Autodesk Inventor part; units mm, degrees
ref_plane "YZ Plane" through (0, 0, 0) normal (1, 0, 0) x (0, 1, 0)
ref_plane "XZ Plane" through (0, 0, 0) normal (0, 1, 0) x (-1, 0, 0)
ref_plane "XY Plane" through (0, 0, 0) normal (0, 0, 1) x (1, 0, 0)
sketch "スケッチ1" plane through (0, 0, 0) normal (0, 0, 1) x (1, 0, 0)
  circle A0 centre (-137.47813, 108.715013) radius 1.5
  circle A1 centre (-137.47813, 108.715013) radius 4
  circle A2 centre (-84.833891, 108.084965) radius 1.5
  circle A3 centre (-84.833891, 108.084965) radius 4
  arc A4 (-118.947299, 71.123436) -> (-117.73095, 71.382243) centre (-118.502117, 72.018876) ccw
  arc A5 (-114.600271, 73.907195) -> (-117.73095, 71.382243) centre (-110, 65) ccw
  arc A6 (-114.600271, 73.907195) -> (-114.089743, 75.041147) centre (-115.059151, 74.795694) ccw
  line L0 (-114.089743, 75.041147) -> (-119.33341, 95.750821)
  arc A7 (-119.33341, 95.750821) -> (-120.080809, 96.480412) centre (-120.302818, 95.505368) ccw
  arc A8 (-121.730917, 97.23053) -> (-120.080809, 96.480412) centre (-119.081767, 100.868113) ccw
  arc A9 (-121.730917, 97.23053) -> (-122.772044, 97.31398) centre (-122.319616, 96.422178) ccw
  line L1 (-122.772044, 97.31398) -> (-145.176978, 85.94755)
  arc A10 (-145.176978, 85.94755) -> (-145.169733, 84.160308) centre (-144.724551, 85.055748) ccw
  line L2 (-145.169733, 84.160308) -> (-118.947299, 71.123436)
  arc A11 (-111.181518, 75.777506) -> (-110.19287, 75.023145) centre (-110.212109, 76.022959) ccw
  arc A12 (-100.681376, 68.696468) -> (-110.19287, 75.023145) centre (-110, 65) ccw
  arc A13 (-100.681376, 68.696468) -> (-99.603497, 68.076257) centre (-99.751838, 69.065193) ccw
  line L3 (-99.603497, 68.076257) -> (-77.042446, 71.460414)
  arc A14 (-77.042446, 71.460414) -> (-76.670938, 73.303609) centre (-77.190786, 72.449351) ccw
  line L4 (-76.670938, 73.303609) -> (-114.637331, 96.407596)
  arc A15 (-114.637331, 96.407596) -> (-116.126588, 95.307885) centre (-115.15718, 95.553338) ccw
  line L5 (-116.126588, 95.307885) -> (-111.181518, 75.777506)
  circle A16 centre (-150.294817, 85.033166) radius 1.5
  arc A17 (-124.129325, 99.989384) -> (-123.581755, 100.878808) centre (-124.581752, 100.881185) ccw
  arc A18 (-114.594354, 100.531773) -> (-123.581755, 100.878808) centre (-119.081767, 100.868113) ccw
  arc A19 (-114.594354, 100.531773) -> (-114.117, 99.602773) centre (-113.597151, 100.457031) ccw
  line L6 (-114.117, 99.602773) -> (-73.405222, 74.828115)
  arc A20 (-73.405222, 74.828115) -> (-72.36076, 74.831033) centre (-72.885373, 75.682374) ccw
  arc A21 (-73.660486, 68.382589) -> (-72.36076, 74.831033) centre (-70, 71) ccw
  arc A22 (-73.660486, 68.382589) -> (-74.622268, 68.789879) centre (-74.473928, 67.800942) ccw
  line L7 (-74.622268, 68.789879) -> (-99.158476, 65.109447)
  arc A23 (-99.158476, 65.109447) -> (-100.006948, 64.200283) centre (-99.010135, 64.120511) ccw
  arc A24 (-119.754961, 67.311137) -> (-100.006948, 64.200283) centre (-110, 65) ccw
  arc A25 (-119.754961, 67.311137) -> (-120.282843, 68.437115) centre (-120.728025, 67.541674) ccw
  line L8 (-120.282843, 68.437115) -> (-147.085218, 81.762313)
  arc A26 (-147.085218, 81.762313) -> (-148.083283, 81.700131) centre (-147.5304, 80.866873) ccw
  arc A27 (-148.11038, 88.384022) -> (-148.083283, 81.700131) centre (-150.294817, 85.033166) ccw
  arc A28 (-148.11038, 88.384022) -> (-147.111844, 88.329935) centre (-147.564271, 89.221736) ccw
  line L9 (-147.111844, 88.329935) -> (-124.129325, 99.989384)
  circle A29 centre (-110, 65) radius 7.025
  circle A30 centre (-119.081767, 100.868113) radius 1.5
  circle A31 centre (-70, 71) radius 1.5
  line L10 (-330.399972, 95) -> (-110, 65)
  circle A32 centre (-156.443214, 91.162336) radius 4
  circle A33 centre (-136.470623, 92.209055) radius 4
  line L11 (0, 0) -> (-155.794817, 0)
  line L12 (-329.051247, 104.90863) -> (-108.651275, 74.90863)
  circle A34 centre (-156.443214, 91.162336) radius 9
  circle A35 centre (-136.470623, 92.209055) radius 6
  line L13 (-156.443214, 91.162336) -> (-136.470623, 92.209055)
  circle A36 centre (-110, 65) radius 65
  circle A37 centre (-191.443214, 91.162336) radius 5
  line L14 (-191.443214, 91.162336) -> (-156.443214, 91.162336)
  line L15 (-191.443214, 91.162336) -> (-206.443214, 91.162336)
  circle A38 centre (-206.443214, 91.162336) radius 5
  line L16 (-206.443214, 91.162336) -> (-221.443214, 91.162336)
  circle A39 centre (-221.443214, 91.162336) radius 5
  line L17 (-221.443214, 91.162336) -> (-236.443214, 91.162336)
  circle A40 centre (-236.443214, 91.162336) radius 5
  line L18 (-206.843214, 96.14631) -> (-157.163214, 100.133489)
  line L19 (-206.843214, 86.178361) -> (-157.163214, 82.191182)
  line L20 (-135.882319, 98.180143) -> (-155.560758, 100.118968)
  line L21 (-154.629369, 82.34701) -> (-135.261393, 86.332171)
  circle A41 centre (-206.443214, 91.162336) radius 1.5
  circle A42 centre (-191.443214, 91.162336) radius 1.5
  line L22 (-236.443214, 91.162336) -> (-191.443214, 91.162336) construction
  line L23 (-236.443214, 86.162336) -> (-191.443214, 86.162336)
  line L24 (-191.443214, 96.162336) -> (-236.443214, 96.162336)
  arc A43 (-236.443214, 96.162336) -> (-236.443214, 86.162336) centre (-236.443214, 91.162336) ccw
  arc A44 (-191.443214, 86.162336) -> (-191.443214, 96.162336) centre (-191.443214, 91.162336) ccw
  point P0 (-202.811763, 87.725395)
  point P1 (-169.324077, 83.167179)
  point P2 (-153.510113, 82.653698)
  point P3 (-153.460125, 82.587594)
  point P4 (-191.336809, 86.163468)
  point P5 (-192.881846, 86.373772)
  point P6 (-213.943214, 91.162336)
  dimension "d0" = 8
  dimension "d1" = 8
  dimension "d2" = 95
  dimension "d3" = 7.75125
  dimension "d4" = 10
  dimension "d5" = 18
  dimension "d6" = 12
  dimension "d7" = 20
  dimension "d8" = 3
  dimension "d9" = 130
  dimension "d10" = 10
  dimension "d11" = 35
  dimension "d12" = 15
  dimension "d13" = 10
  dimension "d14" = 15
  dimension "d15" = 10
  dimension "d16" = 15
  dimension "d17" = 10
  dimension "d18" = 3
  dimension "d19" = 3
  dimension "d20" = 10
extrude "押し出し1" add sketch "スケッチ1" against normal blind 5 contours A37 L12 | L12 A37 L15 A42 L14 | L23 A39 L12 A38 L19 | L19 A38 L23 | A37 L23 A38 L12 | L12 A38 L15 A37 | L14 A42 L15 A37 | A38 L12 | L23 A40 L17 L12 A39 | A39 L12 | L12 A38 L16 A41 L15 | L15 A38 L24 A37 | A42 L15 L14 | L14 L15 A42 | L24 A38 L18 | L18 A38 L16 A39 L24 | L12 A39 L16 A38 | A39 L17 L16 L12 | L12 L17 A39 | A40 L12 | L15 A41 L16 A38 | A39 L16 L17 | A39 L17 L12 A40 L24 | L17 A40 L12 | A40 L12 | A41 L16 L15 | L15 L16 A41
hole "穴1" at (-236.443214, 91.162336, 0) at (-221.443214, 91.162336, 0) at (-206.443214, 91.162336, 0) at (-191.443214, 91.162336, 0) direction (0, 0, -1) diameter 3 depth 12 tip angle 118
properties part number "カウンター 取り付け根元延長"
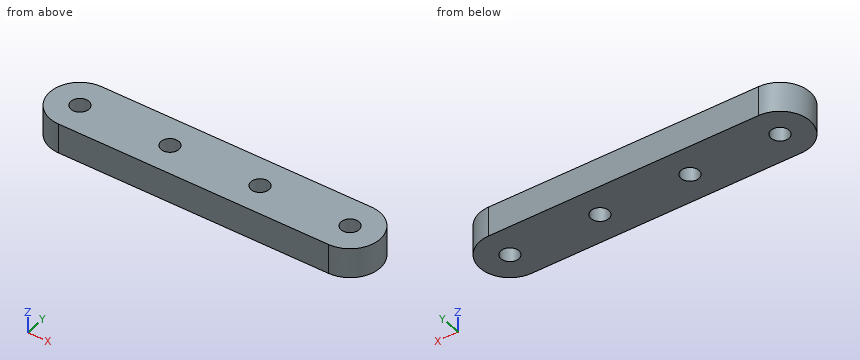
Can you work these out from the model? Positions are in its coordinate system, mm. Round coordinates to 2 decimals unless told otherwise and drop trailing zeros. Order: outer loops, then holes, each group sorted by start corner. A loop starts at its lowest first (then second) coordinate and runs counter-clockwise, first axis right, second up. Notation, with made-up numbers: (62, 48.5) -> (74, 48.5) arc R27 ccw to (74, 64.5) -> close; hole circle Ø5 at (4.5, 50.25). An arc over 180 degrees is marked (long way). Return JSON: item names as keys, results as strings. Group by question number.
1. If we section it at B-B, the plane z = -3.05: Write out the boundary of the cut face in (x, y).
2. If we section it at D-D, the plane y = 94.75: Write out the boundary of the cut face in (x, z), then the cut area to 3 significant figures.
3. Will these pins go through, and if not, where does the flat tip stop? pin 1 (2.5 mm diameter, centred on x = -221.44, y = 91.16, fed in from -Z); pin 2 (1 mm diameter, centred on y = 89.5, z = -2, fed in from -X).
4. If we section it at C-C, the plane y = 87.75: Write out the boundary of the cut face in (x, z).
5. I need wall thicknesses on line 1 (X direction, y = 92, z = -3.4); line 2 (X direction, y = 90.25, z = -1.3); line 3 (Y direction, x = -206.5, z = -3.1). Which ranges of each line are inside material? Lowest first, please. Write a range as [from, to].
6. If we section it at A-A, the plane x = -222: Write out the boundary of the cut face in (y, z).
Output values:
{
 "1": {"outline": "(-236.44, 86.16) -> (-191.44, 86.16) arc R5 ccw to (-191.44, 96.16) -> (-236.44, 96.16) arc R5 ccw to start; hole circle Ø3 at (-236.44, 91.16); hole circle Ø3 at (-221.44, 91.16); hole circle Ø3 at (-206.44, 91.16); hole circle Ø3 at (-191.44, 91.16)"},
 "2": {"outline": "(-239.93, -5) -> (-187.96, -5) -> (-187.96, 0) -> (-239.93, 0) -> close", "area": "260 mm²"},
 "3": {"pin 1": "through", "pin 2": "x = -241.31"},
 "4": {"outline": "(-240.1, -5) -> (-187.79, -5) -> (-187.79, 0) -> (-240.1, 0) -> close"},
 "5": {"line 1": "[-241.37, -237.69], [-235.2, -222.69], [-220.2, -207.69], [-205.2, -192.69], [-190.2, -186.51]", "line 2": "[-241.36, -237.63], [-235.25, -222.63], [-220.25, -207.63], [-205.25, -192.63], [-190.25, -186.53]", "line 3": "[86.16, 89.66], [92.66, 96.16]"},
 "6": {"outline": "(86.16, -5) -> (89.77, -5) -> (89.77, 0) -> (86.16, 0) -> close; (92.56, -5) -> (96.16, -5) -> (96.16, 0) -> (92.56, 0) -> close"}
}
